Input: part model. Units: mm. Frame: model coordinates. Coordinates: 2 decimals unless noted, no trailing zeros. Order: outer loops, then holes, each group sorted by start corner. A loop starts at its lowest first (then second) coordinate and runs counter-clockwise, first axis right, second up.
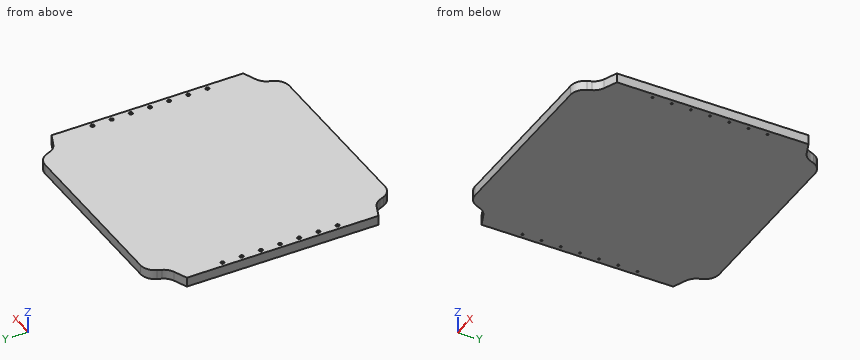
from build123d import *

# Parameters (mm, degrees)
BOSS_EXTRUDE1_DEPTH                                = 25.4
FILLET1_R                                          = 38.1
CSK_FOR_10_FLAT_HEAD_MACHINE_SCREW_100_D           = 5.1054
CSK_FOR_10_FLAT_HEAD_MACHINE_SCREW_100_CSINK_D     = 9.779
CSK_FOR_10_FLAT_HEAD_MACHINE_SCREW_100_CSINK_ANGLE = 100


with BuildPart() as part:
    # Sketch1 → Boss-Extrude1 (new body)
    with BuildSketch(Plane.XY):
        Polygon((-254, 0), (254, 0), (274.458591334, 49.391408666), (323.85, 69.85), (323.85, 577.85), (274.458591334, 598.308591334), (254, 647.7), (-254, 647.7), (-274.458591334, 598.308591334), (-323.85, 577.85), (-323.85, 69.85), (-274.458591334, 49.391408666), align=None)
    extrude(amount=BOSS_EXTRUDE1_DEPTH)

    # Fillet1
    fillet1_edges = [part.edges().sort_by_distance(p)[0] for p in [
        (254, 0, 12.7),
        (-254, 0, 12.7),
        (-274.458591334, 49.391408666, 12.7),
        (-274.458591334, 598.308591334, 12.7),
        (-254, 647.7, 12.7),
        (254, 647.7, 12.7),
        (274.458591334, 598.308591334, 12.7),
        (274.458591334, 49.391408666, 12.7),
    ]]
    fillet(fillet1_edges, radius=FILLET1_R)

    # CSK for #10 Flat Head Machine Screw (100)1 (through all)
    with Locations(Plane.XY.offset(25.4)):
        with Locations((311.15, 323.85), (311.15, 374.65), (311.15, 425.45), (311.15, 273.05), (311.15, 222.25), (311.15, 171.45), (311.15, 476.25)):
            csk_for_10_flat_head_machine_screw_100 = CounterSinkHole(CSK_FOR_10_FLAT_HEAD_MACHINE_SCREW_100_D / 2, CSK_FOR_10_FLAT_HEAD_MACHINE_SCREW_100_CSINK_D / 2, counter_sink_angle=CSK_FOR_10_FLAT_HEAD_MACHINE_SCREW_100_CSINK_ANGLE)

    # Mirror1: CSK for #10 Flat Head Machine Screw (100)1 across plane
    add(csk_for_10_flat_head_machine_screw_100.mirror(Plane(origin=(0, 0, 0), x_dir=(0, 0, 1), z_dir=(1, 0, 0))), mode=Mode.SUBTRACT)


solid = part.part
Item 1: Ray query, probe 1 along X at (y, z) = (323.85, 10); probe 2 along X at (y, z) = (595, 11); probe 3 along X at (y, z) = (583, 21.75). Return the intervals inside material, ascending.
Response values:
probe 1: x = -323.85 to -313.7, -308.6 to 308.6, 313.7 to 323.85
probe 2: x = -283.68 to 283.68
probe 3: x = -311.42 to 311.42
Item 2: Pin query (flat end, axial travel): pin 1 Ø4 at (x, y) = (311.15, 222.25) entering from +Z; pin 2 Ø6 at (x, y) = (-311.15, 323.85) entering from +Z; pin 3 Ø6.5 at (x, y) = (-311.15, 273.05) entering from +Z; pin 4 Ø8 at (x, y) = (311.15, 323.85) entering from +Z. Return the tip coordinate at first contact, or that it passes through.
Response values:
pin 1: passes through
pin 2: stops at z = 23.81
pin 3: stops at z = 24.02
pin 4: stops at z = 24.65
Item 3: Cut plane A-A on z = 12.5. Count the separate pieces of the cut face and the enclosed holes in it, then the cut area to 3 significant figures.
Response values:
separate pieces: 1
enclosed holes: 14
area: 405,000 mm2
Item 4: Cut plane B-B on x = -249.5. Return loops of the section in (y, z), then the cut area to 3 significant figures.
Response values:
outline: (6.28, 0) - (641.42, 0) - (641.42, 25.4) - (6.28, 25.4) - close
area: 16,100 mm2
